```python
from build123d import *

# Parameters (mm, degrees)
BASE_PLATE_R        = 1.6
EXTRUDE_1_DEPTH     = 6
CUT_EXTRUDE_START   = -6
SKETCH_1_R          = 3.25
SKETCH_1_R_2        = 3.5
CUT_EXTRUDE_1_DEPTH = 4.5
SKETCH_1_6_R        = 2.4
CUT_EXTRUDE_2_DEPTH = 2
SKETCH_1_7_R        = 2.5
CUT_EXTRUDE_3_DEPTH = 1.4
FILLET_2_R          = 0.5
CHAMFER_1_SIZE      = 0.4


with BuildPart() as part:
    # Base plate → 凸台-拉伸1 (new body)
    with BuildSketch(Plane(origin=(0, 0, 0), x_dir=(1, 0, 0), z_dir=(0, 1, 0))):
        with BuildLine():
            ThreePointArc((-38.1, -33.9), (-36.869848481, -36.869848481), (-33.9, -38.1))
            Line((-33.9, -38.1), (33.9, -38.1))
            ThreePointArc((33.9, -38.1), (36.869848481, -36.869848481), (38.1, -33.9))
            Line((38.1, -33.9), (38.1, 33.9))
            ThreePointArc((38.1, 33.9), (36.869848481, 36.869848481), (33.9, 38.1))
            Line((33.9, 38.1), (-0.9, 38.1))
            Line((-0.9, 38.1), (-0.9, 27.4))
            ThreePointArc((-0.9, 27.4), (-2.9, 25.4), (-4.9, 27.4))
            Line((-4.9, 27.4), (-4.9, 38.1))
            Line((-4.9, 38.1), (-33.9, 38.1))
            ThreePointArc((-33.9, 38.1), (-36.869848481, 36.869848481), (-38.1, 33.9))
            Line((-38.1, 33.9), (-38.1, -33.9))
        make_face()
        with Locations(Location((-33.9, -33.9, 0), (0, 0, 270))):
            Circle(BASE_PLATE_R, mode=Mode.SUBTRACT)
        with Locations(Location((33.9, -33.9, 0), (0, 0, 270))):
            Circle(BASE_PLATE_R, mode=Mode.SUBTRACT)
        with Locations(Location((-33.9, 33.9, 0), (0, 0, 270))):
            Circle(BASE_PLATE_R, mode=Mode.SUBTRACT)
        with Locations(Location((33.9, 33.9, 0), (0, 0, 270))):
            Circle(BASE_PLATE_R, mode=Mode.SUBTRACT)
    extrude(amount=EXTRUDE_1_DEPTH)

    # 草图1 → 切除-拉伸1 (cut)
    with BuildSketch(Plane.XZ.offset(CUT_EXTRUDE_START)):
        with Locations(Location((-0.35, 10.415, 0), (0, 0, 90))):
            Circle(SKETCH_1_R)
        with Locations(Location((-22.7, 23.9, 0), (0, 0, 90))):
            Circle(SKETCH_1_R)
        with Locations(Location((-22.7, -3.07, 0), (0, 0, 90))):
            Circle(SKETCH_1_R)
        with Locations(Location((-17.96, -15.36, 0), (0, 0, 90))):
            Circle(SKETCH_1_R_2)
        with Locations(Location((-5.01, -15.36, 0), (0, 0, 90))):
            Circle(SKETCH_1_R_2)
    extrude(amount=CUT_EXTRUDE_1_DEPTH, mode=Mode.SUBTRACT)

    # 草图1<6> → 切除-拉伸2 (cut)
    with BuildSketch(Plane.XZ.offset(CUT_EXTRUDE_START)):
        with BuildLine():
            Line((8.9, 2), (8.9, -7.4))
            ThreePointArc((8.9, -7.4), (11.4, -9.9), (13.9, -7.4))
            Line((13.9, -7.4), (13.9, 2))
            ThreePointArc((13.9, 2), (11.4, 4.5), (8.9, 2))
        make_face()
        with BuildLine():
            Line((21.6, -0.16), (21.6, -5.24))
            ThreePointArc((21.6, -5.24), (24.1, -7.74), (26.6, -5.24))
            Line((26.6, -5.24), (26.6, -0.16))
            ThreePointArc((26.6, -0.16), (24.1, 2.34), (21.6, -0.16))
        make_face()
        with Locations(Location((31.9, -15.1, 0), (0, 0, 90))):
            Circle(SKETCH_1_6_R)
        with Locations(Location((16.7, -15.1, 0), (0, 0, 90))):
            Circle(SKETCH_1_6_R)
    extrude(amount=CUT_EXTRUDE_2_DEPTH, mode=Mode.SUBTRACT)

    # 草图1<7> → 切除-拉伸3 (cut)
    with BuildSketch(Plane.XZ.offset(CUT_EXTRUDE_START)):
        with BuildLine():
            Line((21.65, -38.1), (21.65, -37.1))
            Line((21.65, -37.1), (21.65, -36.1))
            ThreePointArc((21.65, -36.1), (20.560909108, -34.172620939), (18.347964405, -34.111100529))
            ThreePointArc((18.347964405, -34.111100529), (17.472620939, -34.939090892), (17.15, -36.1))
            Line((17.15, -36.1), (17.15, -38.1))
            Line((17.15, -38.1), (21.65, -38.1))
        make_face()
        with BuildLine():
            Line((21.65, -37.1), (25.452035595, -35.088899471))
            ThreePointArc((25.452035595, -35.088899471), (23.239090892, -35.027379061), (22.15, -33.1))
            Line((22.15, -33.1), (22.15, -32.1))
            Line((22.15, -32.1), (18.347964405, -34.111100529))
            ThreePointArc((18.347964405, -34.111100529), (20.560909108, -34.172620939), (21.65, -36.1))
            Line((21.65, -36.1), (21.65, -37.1))
        make_face()
        with BuildLine():
            ThreePointArc((22.15, -33.1), (24.4, -35.35), (26.65, -33.1))
            Line((26.65, -33.1), (26.65, -28.1))
            ThreePointArc((26.65, -28.1), (24.4, -25.85), (22.15, -28.1))
            Line((22.15, -28.1), (22.15, -33.1))
        make_face()
        with BuildLine():
            ThreePointArc((22.15, -28.1), (23.239090892, -26.172620939), (25.452035595, -26.111100529))
            Line((25.452035595, -26.111100529), (22.211102988, -24.396797462))
            Line((22.211102988, -24.396797462), (21.438912065, -26.051492297))
            ThreePointArc((21.438912065, -26.051492297), (20.115915291, -27.233064766), (18.347964405, -27.088899471))
            Line((18.347964405, -27.088899471), (22.15, -29.1))
            Line((22.15, -29.1), (22.15, -28.1))
        make_face()
        with BuildLine():
            Line((18.761087935, -21.148507703), (17.361087935, -24.148507703))
            ThreePointArc((17.361087935, -24.148507703), (18.448507703, -27.138912065), (21.438912065, -26.051492297))
            Line((21.438912065, -26.051492297), (22.838912065, -23.051492297))
            ThreePointArc((22.838912065, -23.051492297), (21.751492297, -20.061087935), (18.761087935, -21.148507703))
        make_face()
        with BuildLine():
            Line((38.1, -20.6), (30.8, -20.6))
            ThreePointArc((30.8, -20.6), (29.3, -22.1), (30.8, -23.6))
            Line((30.8, -23.6), (38.1, -23.6))
            Line((38.1, -23.6), (38.1, -20.6))
        make_face()
        with BuildLine():
            Line((17.1, 21.71), (17.1, 14.09))
            ThreePointArc((17.1, 14.09), (19.6, 11.59), (22.1, 14.09))
            Line((22.1, 14.09), (22.1, 21.71))
            ThreePointArc((22.1, 21.71), (19.6, 24.21), (17.1, 21.71))
        make_face()
        with Locations(Location((27.7, 17.9, 0), (0, 0, 90))):
            Circle(SKETCH_1_7_R)
    extrude(amount=CUT_EXTRUDE_3_DEPTH, mode=Mode.SUBTRACT)

    # 圆角2
    fillet_2_edges = [part.edges().sort_by_distance(p)[0] for p in [
        (38.1, 5.3, -23.6),
        (38.1, 5.3, -20.6),
        (21.65, 5.3, -38.1),
        (21.65, 5.3, -37.1),
        (22.211102988, 5.3, -24.396797462),
        (22.15, 5.3, -29.1),
        (22.15, 5.3, -32.1),
        (17.15, 5.3, -38.1),
    ]]
    fillet(fillet_2_edges, radius=FILLET_2_R)

    # 倒角1
    chamfer_1_edges = [part.edges().sort_by_distance(p)[0] for p in [
        (29.3, 6, -22.1),
        (22.1, 6, 17.9),
        (19.6, 6, 11.59),
        (17.1, 6, 17.9),
        (19.6, 6, 24.21),
        (27.7, 6, 15.4),
        (26.65, 6, -30.6),
        (17.472620939, 6, -34.939090892),
        (17.266935234, 6, -25.815915291),
        (18.061087935, 6, -22.648507703),
        (21.751492297, 6, -20.061087935),
        (26.327379061, 6, -26.939090892),
        (26.327379061, 6, -34.260909108),
        (28.025, 6, -38.1),
        (34.2, 6, -20.6),
        (34.2, 6, -23.6),
        (38.1, 6, -29),
        (21.65, 6, -37.500581317),
        (23.684124954, 6, -36.024042222),
        (24.041794054, 6, -25.365148146),
        (22.625579348, 6, -23.508633834),
        (20.115875046, 6, -28.024042222),
        (22.15, 6, -30.6),
        (20.115875046, 6, -33.175957778),
        (17.15, 6, -36.85),
        (22.391323808, 6, -24.336310391),
        (22.078306458, 6, -29.143182832),
        (22.078306458, 6, -32.056817168),
        (21.721693542, 6, -37.143182832),
        (37.953553391, 6, -20.453553391),
        (37.953553391, 6, -23.746446609),
        (17.003553391, 6, -37.953553391),
        (21.796446609, 6, -37.953553391),
        (-19.4, 6, -38.1),
        (-36.869848481, 6, -36.869848481),
        (-38.1, 6, 0),
        (-36.869848481, 6, 36.869848481),
        (0, 6, 38.1),
        (36.869848481, 6, 36.869848481),
        (38.1, 6, 6.9),
        (36.869848481, 6, -36.869848481),
        (-5.01, 6, -18.86),
        (-17.96, 6, -18.86),
        (-22.7, 6, -6.32),
        (7.875, 6, -38.1),
        (-22.7, 6, 20.65),
        (-0.35, 6, 7.165),
        (13.9, 6, -2.7),
        (11.4, 6, -9.9),
        (8.9, 6, -2.7),
        (11.4, 6, 4.5),
        (26.6, 6, -2.7),
        (24.1, 6, -7.74),
        (21.6, 6, -2.7),
        (24.1, 6, 2.34),
        (31.9, 6, -17.5),
        (16.7, 6, -17.5),
    ]]
    chamfer(chamfer_1_edges, length=CHAMFER_1_SIZE)


solid = part.part
```
Verification items for the finished model (mm, model axes). A direction names the side the tool comes from. Round coordinates to 2 decimals unless told otherwise and drop trailing zeros. Write each loop counter-clockwise with the first axis right and the second up, starting at its lowest first coordinate (ties: lowest second). Pieces come first, ordered by that corner, then holes. Notation, with made-up numbers: (-9.5, 68) - (4.5, 68) arc R21 ccw to (4.5, 85) - close; hole circle Ø8 at (-2, 43). An arc over 180 degrees is marked (long way). Answer as a JSON object with one key per item and string values. Group by question number.
Q1. Go/stop test with a flat-tipped pin: pin 1 Ø4.5 at (x, z) = (16.7, -15.1) entering from +Y. Record where the tip stops, or that it passes through.
Q2. Thickness scan on line 1 (X direction, y = 4.75, z = -15.1); line 2 (X direction, y = 4.4, z = -33.9); line 3 (X direction, y = 2.9, z = -3.07). Record the ranges inside material, lowest first.
Q3. Mould release check, pull along Z, two halves, no side actions. Record for faces 3 (the conical face through (-36.637, 5.886, -36.698)), 4 (the flat face through (-1, 6, -1)), 5 (the flat face through (-23, 1.5, 24)): released by +Z, released by -Z, zero draft, split by the parting line, or undercut.
Q4. Section check A-A, the plane x = -17.96. Enter the section's corners in (y, z), plus the area to 3 significant figures.
Q5. Tool access check on faces 1 (the conical face through (-36.698, 5.886, 36.637)), 2 (the flat face through (20, 5.8, -28.19)). Record the directions out of +Z, -Z, +X, -X, +Y, -Y that give a thin tool (end or side, any length) a straight path to the whole face; none if there is none.
Found:
{
 "1": {"pin 1": "stops at y = 4"},
 "2": {"line 1": "x = -38.1 to -21.45, -14.47 to -8.5, -1.52 to 14.3, 19.1 to 29.5, 34.3 to 38.1", "line 2": "x = -38.1 to -35.5, -32.3 to -4.9, -0.9 to 32.3, 35.5 to 38.1", "line 3": "x = -38.1 to -25.95, -19.45 to 38.1"},
 "3": {"face 3": "released by -Z", "face 4": "zero draft", "face 5": "undercut"},
 "4": {"outline": "(0, -38.1) - (5.6, -38.1) - (6, -37.7) - (6, -19.26) - (5.6, -18.86) - (1.5, -18.86) - (1.5, -11.86) - (5.6, -11.86) - (6, -11.46) - (6, 37.7) - (5.6, 38.1) - (0, 38.1) - close", "area": "425 mm^2"},
 "5": {"face 1": "+Z, -X, +Y", "face 2": "+Y"}
}
